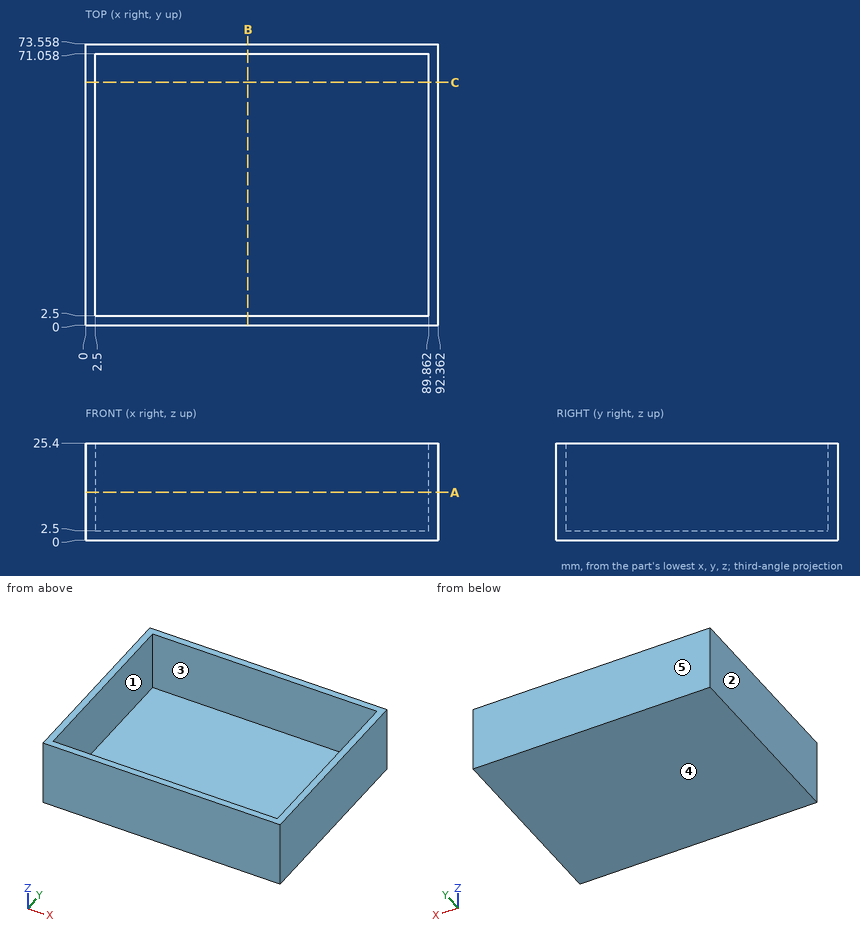
Verification items for this drawing (mm, ordinates from the low corner). A direction names the side the tool comes from. Round coordinates to 2 decimals unless told otherwise and drop trailing zeros. Loops run counter-clockwise (first coordinate to the right, second up) from the corner with the lowest first, then second, coordinate; pieces in that order, holes last. Notation, with made-up numbers: (55.5, 36.5) - (73.5, 36.5) arc R11 ccw to (73.5, 54.5) - close; hole circle Ø3 at (49, 44). An arc over 180 degrees is marked (long way). Write item = value, one per line.
Q1. Mould release check, pull along Y, two halves, no side actions. Record for the marked faces 3, 4 and 5: +Y half, -Y half, draft (parallel to the pull), parting line (faces both ways), or undercut.
Here are the results:
face_3 = undercut
face_4 = draft
face_5 = +Y half
Q2. Sectioned sample at A-A on z = 12.5. Record the boundary of the cut face in (x, y).
Here are the results:
outline = (0, 0) - (92.36, 0) - (92.36, 73.56) - (0, 73.56) - close; hole (2.5, 2.5) - (89.86, 2.5) - (89.86, 71.06) - (2.5, 71.06) - close
Q3. Tool access check on the marked faces 1 and 2. Record the directions out of +Z, -Z, +X, -X, +Y, -Y that give a thin tool (end or side, any length) a straight path to the whole face; none if there is none.
Here are the results:
face_1 = +Z
face_2 = +Z, -Z, -X, +Y, -Y
Q4. Sectioned sample at C-C on y = 63.5. Record the boundary of the cut face in (x, z).
Here are the results:
outline = (0, 0) - (92.36, 0) - (92.36, 25.4) - (89.86, 25.4) - (89.86, 2.5) - (2.5, 2.5) - (2.5, 25.4) - (0, 25.4) - close
Q5. Material ranges on L1, parallel to Y at x = 80.5, z = 8; L2, parallel to X at y = 6, z = 21.5; L3, parallel to Z at x = 9.5, y = 6.5, recorded low to high.
Here are the results:
L1 = 0 to 2.5, 71.06 to 73.56
L2 = 0 to 2.5, 89.86 to 92.36
L3 = 0 to 2.5
Q6. Sectioned sample at B-B on x = 42.5. Record the boundary of the cut face in (y, z).
Here are the results:
outline = (0, 0) - (73.56, 0) - (73.56, 25.4) - (71.06, 25.4) - (71.06, 2.5) - (2.5, 2.5) - (2.5, 25.4) - (0, 25.4) - close
Q7. Depth check by flat-ended pin: pin 1 (6 mm diameter, centred on x = 23, y = 57.5, fed in from +Z). Enter the tip coordinate at first touch or a pass-through.
Here are the results:
pin_1 = 2.5
